```python
from build123d import *

# Parameters (mm, degrees)
F1_DEPTH = 12
F2_DEPTH = 2
F3_R     = 1.49999


# Not quite as in the source:
# - a fillet or chamfer is up to 0.001 mm smaller than in the source, because OpenCascade refuses the exact size


with BuildPart() as f1:
    # F0 (on Top) → F1 (new body)
    with BuildSketch(Plane.XY):
        with BuildLine():
            ThreePointArc((-0.5, -2.1937410968), (-2.25, 0), (-0.5, 2.1937410968))
            Line((-0.5, 2.1937410968), (-0.5, 5.853684737))
            ThreePointArc((-0.5, 5.853684737), (-5.875, 0), (-0.5, -5.853684737))
            Line((-0.5, -5.853684737), (-0.5, -2.1937410968))
        make_face()
    extrude(amount=F1_DEPTH)

    # F0 (on Top) → F2 (join)
    with BuildSketch(Plane.XY):
        with BuildLine():
            ThreePointArc((-0.5, -5.853684737), (-5.875, 0), (-0.5, 5.853684737))
            Line((-0.5, 5.853684737), (-0.5, 8.8609042992))
            ThreePointArc((-0.5, 8.8609042992), (-8.875, 0), (-0.5, -8.8609042992))
            Line((-0.5, -8.8609042992), (-0.5, -5.853684737))
        make_face()
    extrude(amount=F2_DEPTH)

    # F3 (radius 1.5 in the source; OpenCascade refuses exactly that, so slightly less here)
    f3_edges = [f1.edges().sort_by_distance(p)[0] for p in [
        (-5.875, 0, 2),
        (-8.875, 0, 2),
        (-5.875, 0, 12),
        (-2.25, 0, 12),
    ]]
    fillet(f3_edges, radius=F3_R)


solid = f1.part
```
Geometry check sheet. Reference: the model listing, model coordinates, mm. Coordinates: 2 decimals unless noted, no trailing zeros. Write each loop counter-clockwise with the first axis right and the second up, starting at its lowest first coordinate (ties: lowest second). Pieces come first, ordered by that corner, then holes. Notation, with made-up numbers: M -33,75 L 8,75 A33 cw 8,104 Z; hole C 17,20 d2. An arc over 180 degrees is marked long. Use one line per item in the form item = value. Start each with the question number.
1) Go/stop test with flat-tipped pins: pin 1 Ø5 at (x, z) = (-6, 10) entering from -Y; pin 2 Ø4 at (y, z) = (-4, 6.5) entering from -X. Record where each tip stops, or that it passes through.
2) Thickness scan on probe 1 along Y at (x, z) = (-2, 5.75); probe 2 along Z at (x, y) = (-6, 1); probe 3 along Y at (x, z) = (-3.5, 10.25). Record the ranges inside material, lowest first. Write a range as from..to.
3) Section check A-A on z = 9.5. Enter the section's corners in (x, y) (3 decimals), and give its area (3 significant figures).
4) Section check B-B on z = 2.5. Enter the section's corners in (x, y), and give its area (3 significant figures).
5) Release check for a two-part mould opening along Y. For faces 1 (the cylindrical face through (-2.25, -0.04, 5.18)), 2 (the cylindrical face through (-5.874, 0.122, 6.951)), 3 (the flat face through (-4, 0, 12)) record: pulls with the +Y half, pulls with the -Y half, needs draft (parallel to the pull), parting line crosses it, or undercut.
Responses:
q1.pin_1 = -4.72
q1.pin_2 = -5.52
q2.probe_1 = -5.52..-1.03, 1.03..5.52
q2.probe_2 = 0..2.74
q2.probe_3 = -4.72..4.72
q3.outline = M -0.5,-5.854 L -0.5,-2.194 A2.25 cw -0.5,2.194 L -0.5,5.854 A5.875 ccw Z
q3.area = 42.6 mm2
q4.outline = M -0.5,-6.24 L -0.5,-2.19 A2.25 cw -0.5,2.19 L -0.5,6.24 A6.26 ccw Z
q4.area = 49.5 mm2
q5.face_1 = undercut
q5.face_2 = parting line crosses it
q5.face_3 = needs draft
